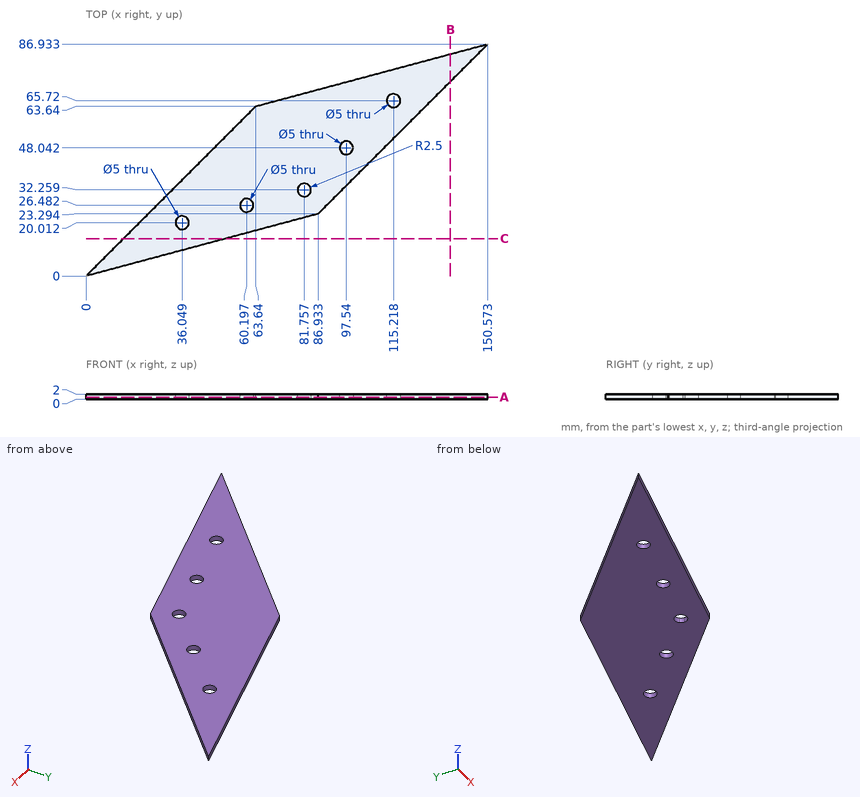
Geometry: see drawing. Coordinates: mm, zero at the bounding-box minimum. Coordinates: 2 decimals unless noted, no trailing zeros. Loops run counter-clockwise (first coordinate to the right, second up) from the corner with the lowest first, then second, coordinate; pieces in that order, holes last. Notation, with made-up numbers: M 17,17 L 29,17 A9 ccw 29,24 Z; hole C 51.5,31 d7. An arc over 180 degrees is marked long. Put each result on its own line as item: value. Start each with the question number.
1) Cut plane B-B on x = 136.5. Return the cut outline in (y, z).
2) Cut plane A-A on z = 0.85. Return the cut outline in (x, y) (1 decimal).
3) Contact query for flat-ended pins moving along their axis: pin 1 Ø1.5 at (x, y) = (53, 55.5) entering from +Z; pin 2 Ø1 at (x, z) = (42, 1.5) entering from +Y; pin 3 Ø1 at (y, z) = (31.5, 0.5) entering from +X. Output: stop coordinate, or through.
4) Ray query, L1, parallel to X at y = 30, z = 0.85 (1 decimal); L2, parallel to Y at x = 34, z = 1.8 (1 decimal); L3, parallel to X at y = 38, z = 1.05. Return the intervals inside material, ascending. Write a range as from..to.
5) Cut plane C-C on y = 14. Return the cut outline in (x, z).
The answers:
1. outline: M 72.86,0 L 83.16,0 L 83.16,2 L 72.86,2 Z
2. outline: M 0,0 L 86.9,23.3 L 150.6,86.9 L 63.6,63.6 Z; hole C 36,20 d5; hole C 60.2,26.5 d5; hole C 81.8,32.3 d5; hole C 97.5,48 d5; hole C 115.2,65.7 d5
3. pin 1: passes through
3. pin 2: stops at y = 42.5
3. pin 3: stops at x = 95.64
4. L1: x = 30..80.7, 82.8..93.6
4. L2: y = 9.1..18.6, 21.4..34
4. L3: x = 38..101.64
5. outline: M 14,0 L 52.25,0 L 52.25,2 L 14,2 Z
